Part model, mm, in its own coordinate system. A direction names the side the tool comes from. Give positions to 0.01 mm unless a question says otherwise; leave off trailing zeros. Order: outer loops, then holes, each group sorted by start corner. A loop starts at its lowest first (then second) coordinate and runs counter-clockwise, first axis right, second up. Notation, with made-up numbers: (4, 13) - (29, 13) arc R17 cw to (29, 18) - close; hole circle Ø10 at (21, 24). An arc over 180 degrees is marked (long way). Use one line per item in the form item = value. Start each with the question number.
1. Band-saw the part on B-B, the plane x = 4.25. List the corners of the cut face in (y, z), plus the area to 3 significant figures.
2. Band-saw the part on C-C, the plane y = 7.5. List the corners of the cut face in (x, z), plus the area to 3 significant figures.
3. Band-saw the part on D-D, the plane x = 6.5. List the corners of the cut face in (y, z), plus the area to 3 significant figures.
4. Pin check, flat tips, straight feed: P1, Ø1, axis at x = 5, z = -6.5, coming from the -Y side; P2, Ø1.5, axis at x = 6.5, y = 3.5, coming from the +Z side; P3, Ø1.5, axis at x = 4.5, y = 6.5, coming from the +Z side; P4, Ø4, axis at y = 4.5, z = -18.12, coming from the -X side. Stop position of each tip, or through.
5. Tool access for faces 1 (the face through (3, 6, 2)), 2 (the face through (0, 4, -13)), 3 (the face through (5, 5, -25.8)): list every direction of +Z, -Z, +X, -X, +Y, -Y with a clear straight run to the whole face (end or side of a thin tool).
6. Pull direction Z, two halves, no side cores. Call faces 4 (the face through (5, 5, 0)), 5 (the face through (5, 5, -10.44)), 6 (the face through (2.6, 9, -14.9)): +Z half, -Z half, draft (parallel to the pull), parting line (faces both ways), or undercut.
7. Drill centre lines: line 1 (Z direction, x = 4.25, y = 2.5); line 2 (Y direction, x = 8.25, z = -18.12); line 3 (Z direction, x = 8.5, y = 2.25). Where is each one in solid material? Low to high.
8. Band-saw the part on A-A, the plane z = -18.12. List the corners of the cut face in (x, y).
from build123d import *

# Parameters (mm, degrees)
SKETCH1_W             = 3
SKETCH1_H             = 9
BOSS_EXTRUDE1_DEPTH   = 9
BOSS_EXTRUDE1_2_DEPTH = 9
SKETCH2_W             = 9
SKETCH2_H             = 9
BOSS_EXTRUDE2_DEPTH   = 10.44
SKETCH3_W             = 3
SKETCH3_H             = 9
BOSS_EXTRUDE3_DEPTH   = 15.36
SKETCH4_W             = 9
SKETCH4_H             = 9
BOSS_EXTRUDE4_DEPTH   = 9
SKETCH5_R             = 2.5
CUT_EXTRUDE1_DEPTH    = 38.054554376
CUT_EXTRUDE5_DEPTH    = 38.054554376


with BuildPart() as part:
    # Sketch1 → Boss-Extrude1 (new body)
    with BuildSketch(Plane.XY):
        with Locations((1.5, 4.5)):
            Rectangle(SKETCH1_W, SKETCH1_H)
    extrude(amount=BOSS_EXTRUDE1_DEPTH)



with BuildPart() as body_2:
    # Sketch1 → Boss-Extrude1 2 (new body)
    with BuildSketch(Plane.XY):
        with Locations((7.5, 4.5)):
            Rectangle(SKETCH1_W, SKETCH1_H)
    extrude(amount=BOSS_EXTRUDE1_2_DEPTH)


with BuildPart() as part_1:
    add(part.part)

    add(body_2.part)  # Boss-Extrude2 merges body 2
    # Sketch2 → Boss-Extrude2 (add)
    with BuildSketch(Plane(origin=(0, 0, 0), x_dir=(-1, 0, 0), z_dir=(0, 0, -1))):
        with Locations((-4.5, 4.5)):
            Rectangle(SKETCH2_W, SKETCH2_H)
    extrude(amount=BOSS_EXTRUDE2_DEPTH)

    # Sketch3 → Boss-Extrude3 (add)
    with BuildSketch(Plane(origin=(0, 0, -10.44), x_dir=(-1, 0, 0), z_dir=(0, 0, -1))):
        with Locations((-7.5, 4.5)):
            Rectangle(SKETCH3_W, SKETCH3_H)
        with Locations((-1.5, 4.5)):
            Rectangle(SKETCH3_W, SKETCH3_H)
    extrude(amount=BOSS_EXTRUDE3_DEPTH)

    # Sketch4 → Boss-Extrude4 (add)
    with BuildSketch(Plane(origin=(0, 0, -25.8), x_dir=(-1, 0, 0), z_dir=(0, 0, -1))):
        with Locations((-4.5, 4.5)):
            Rectangle(SKETCH4_W, SKETCH4_H)
    extrude(amount=BOSS_EXTRUDE4_DEPTH)

    # Sketch5 → Cut-Extrude1 (cut, through all)
    with BuildSketch(Plane(origin=(9, 0, 0), x_dir=(0, 0, -1), z_dir=(1, 0, 0))):
        with Locations((18.12, 4.5)):
            Circle(SKETCH5_R)
    extrude(amount=-CUT_EXTRUDE1_DEPTH, mode=Mode.SUBTRACT)

    # Sketch6 → Cut-Extrude5 (cut, through all)
    with BuildSketch(Plane(origin=(9, 0, 0), x_dir=(0, 0, -1), z_dir=(1, 0, 0))):
        with BuildLine():
            ThreePointArc((-9, 4.5), (-7.681980515, 7.681980515), (-4.5, 9))
            Line((-4.5, 9), (-9, 9))
            Line((-9, 9), (-9, 4.5))
        make_face()
        with BuildLine():
            ThreePointArc((-4.5, 0), (-7.681980515, 1.318019485), (-9, 4.5))
            Line((-9, 4.5), (-9, 0))
            Line((-9, 0), (-4.5, 0))
        make_face()
        with BuildLine():
            ThreePointArc((-2, 4.5), (-2.732233047, 6.267766953), (-4.5, 7))
            Line((-4.5, 7), (-4.5, 2))
            ThreePointArc((-4.5, 2), (-2.732233047, 2.732233047), (-2, 4.5))
        make_face()
        with BuildLine():
            Line((-4.5, 2), (-4.5, 7))
            ThreePointArc((-4.5, 7), (-7, 4.5), (-4.5, 2))
        make_face()
    extrude(amount=-CUT_EXTRUDE5_DEPTH, mode=Mode.SUBTRACT)


solid = part_1.part
From the geometry:
q1.outline = (0, -34.8) - (9, -34.8) - (9, -25.8) - (0, -25.8) - close; (0, -10.44) - (9, -10.44) - (9, 0) - (0, 0) - close
q1.area = 175 mm²
q2.outline = (0, -34.8) - (9, -34.8) - (9, 7.85) - (6, 7.85) - (6, 0) - (3, 0) - (3, 7.85) - (0, 7.85) - close; hole (3, -25.8) - (6, -25.8) - (6, -10.44) - (3, -10.44) - close
q2.area = 314 mm²
q3.outline = (0, -34.8) - (9, -34.8) - (9, 4.5) arc R4.5 ccw to (0, 4.5) - close; hole circle Ø5 at (4.5, -18.12); hole circle Ø5 at (4.5, 4.5)
q3.area = 346 mm²
q4.P1 = 0
q4.P2 = 8.99
q4.P3 = 0
q4.P4 = through
q5.face_1 = +Z, +Y, -Y
q5.face_2 = +Z, -Z, -X, +Y, -Y
q5.face_3 = +Y, -Y
q6.face_4 = +Z half
q6.face_5 = undercut
q6.face_6 = draft
q7.line_1 = -34.8 to -25.8, -10.44 to 0
q7.line_2 = 0 to 2, 7 to 9
q7.line_3 = -34.8 to -19.21, -17.03 to 3.41, 5.59 to 8.4
q8.outline = (0, 0) - (3, 0) - (3, 2) - (0, 2) - close; (0, 7) - (3, 7) - (3, 9) - (0, 9) - close; (6, 0) - (9, 0) - (9, 2) - (6, 2) - close; (6, 7) - (9, 7) - (9, 9) - (6, 9) - close
